Can you work these out from the drawing? Everything is in mm from the part's minimum corner. Coordinates: 2 decimals unless noted, no trailing zeros. Loops run counter-clockwise (first coordinate to the right, second up) from the corner with the lowest first, then second, coordinate; pieces in that order, holes last. Notation, with made-up numbers: (45, 49.5) -> (102, 49.5) arc R7 ccw to (102, 55.5) -> close; hole circle Ø6 at (37, 22.25). An arc over 180 degrees is marked (long way). Use one line per item in the form item = value. Start each with the question number.
(1) Imagine slicing it at B-B (y = 8). List the corners of the cut face in (x, z) for me, plus the area to 3 significant figures.
(2) I need wall thicknesses on line 1 (Y direction, x = 6, z = 5); line 2 (Y direction, x = 3.5, z = 3.75); line 3 (X direction, y = 4.5, z = 6). Which ranges of each line are inside material? Lowest first, please. Write a range as [from, to].
(3) Imagine slicing it at A-A (x = 5). List the corners of the cut face in (y, z) for me.
(4) Thinking about a two-plate mould opening in Z: for the marked faces 1, 2 and 3, which applies, released by +Z, released by -Z, zero draft, split by the parting line, or undercut?
(5) I'm going to push flat-ended pins straight in: pin 1 (4 mm diameter, centred on x = 7.5, z = 6, fed in from +Y); pin 2 (2 mm diameter, centred on x = 3, y = 4, fed in from +Z); pin 3 (2 mm diameter, centred on y = 7.5, z = 3, fed in from -X); pin 4 (5 mm diameter, centred on y = 12.5, z = 2.5, fed in from +X). Where does each tip first touch, or does it pass through?
(6) Imagine slicing it at D-D (y = 10.75). List the corners of the cut face in (x, z) for me.
(7) Imagine slicing it at C-C (y = 2). List the corners of the cut face in (x, z) for me, plus the area to 3 significant figures.
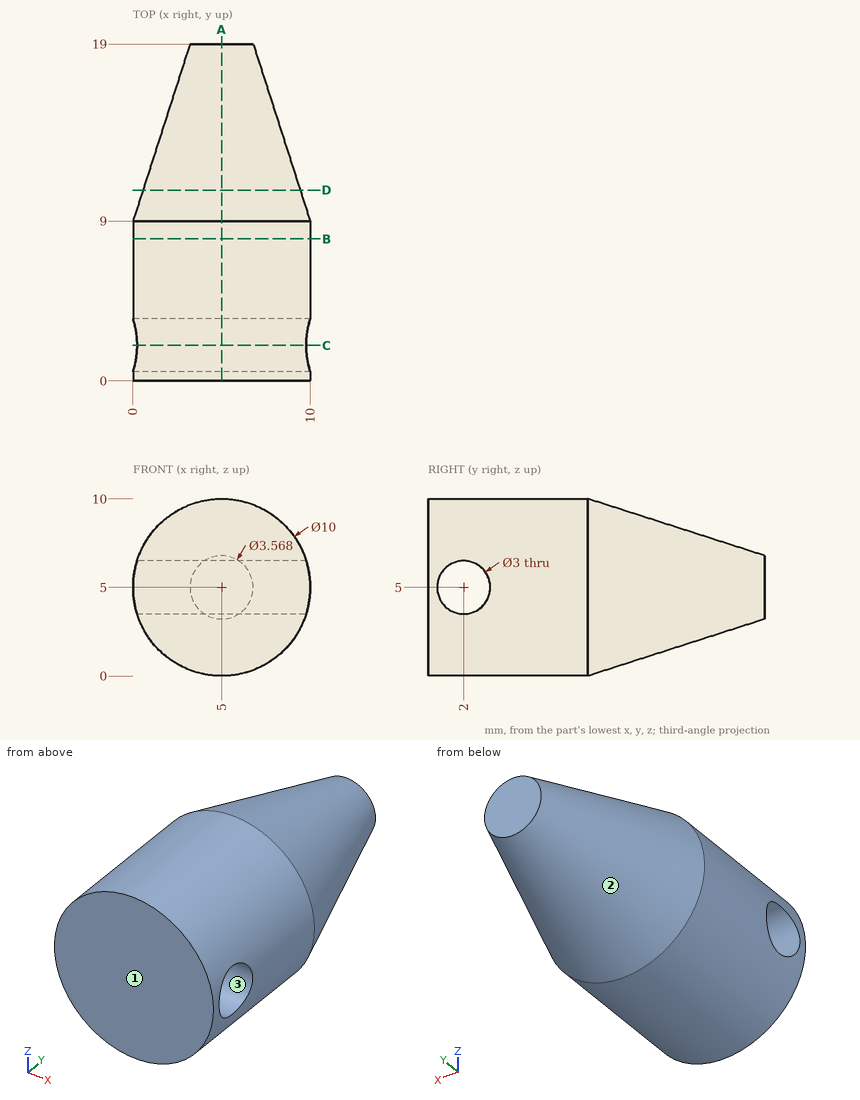
Worked out:
q1.outline = circle Ø10 at (5, 5)
q1.area = 78.5 mm2
q2.line_1 = [0, 0.5], [3.5, 19]
q2.line_2 = [0, 1.17], [2.83, 18.48]
q2.line_3 = [0.1, 9.9]
q3.outline = (0, 0) -> (9, 0) -> (19, 3.22) -> (19, 6.78) -> (9, 10) -> (0, 10) -> close; hole circle Ø3 at (2, 5)
q4.face_1 = zero draft
q4.face_2 = split by the parting line
q4.face_3 = undercut
q5.pin_1 = 19
q5.pin_2 = 9.9
q5.pin_3 = 0.1
q5.pin_4 = 9.41
q6.outline = circle Ø8.87 at (5, 5)
q7.outline = (0.23, 3.5) arc R5 ccw to (9.77, 3.5) -> close; (0.23, 6.5) -> (9.77, 6.5) arc R5 ccw to start
q7.area = 49.0 mm2
